Model file for the job. Use its own axes, mm. A direction names the side the tool comes from. Give positions to 0.01 mm unless a question says otherwise; leave off trailing zeros. Loops run counter-clockwise (first coordinate to the right, second up) from the corner with the lowest first, then second, coordinate; pieces in that order, holes last. Notation, with made-up numbers: (-31.75, 42.25) - (-13.75, 42.25) arc R32 ccw to (-13.75, 79.25) - close; hole circle Ø10 at (75.5, 13). An arc over 180 degrees is marked (long way). Use a Markdown table: item, result.
from build123d import *

# Parameters (mm, degrees)
SKETCH1_W           = 57.15
SKETCH1_H           = 57.15
SKETCH1_W_2         = 44.45
SKETCH1_H_2         = 44.45
BOSS_EXTRUDE1_DEPTH = 457.2
SKETCH2_W           = 44.45
SKETCH2_H           = 6.35
BOSS_EXTRUDE2_DEPTH = 44.45
SKETCH3_R           = 12.7
CUT_EXTRUDE1_DEPTH  = 6.35


with BuildPart() as part:
    # Sketch1 → Boss-Extrude1 (new body)
    with BuildSketch(Plane.XY):
        Rectangle(SKETCH1_W, SKETCH1_H)
        Rectangle(SKETCH1_W_2, SKETCH1_H_2, mode=Mode.SUBTRACT)
    extrude(amount=BOSS_EXTRUDE1_DEPTH)

    # Sketch2 → Boss-Extrude2 (add)
    with BuildSketch(Plane(origin=(0, -22.225, 0), x_dir=(1, 0, 0), z_dir=(0, 1, 0))):
        with Locations((0, -3.175)):
            Rectangle(SKETCH2_W, SKETCH2_H)
    extrude(amount=BOSS_EXTRUDE2_DEPTH)

    # Sketch3 → Cut-Extrude1 (cut)
    with BuildSketch(Plane(origin=(0, 28.575, 0), x_dir=(0, 0, -1), z_dir=(0, 1, 0))):
        with Locations(Location((-25.4, 0, 0), (0, 0, 180))):
            Circle(SKETCH3_R)
    extrude(amount=-CUT_EXTRUDE1_DEPTH, mode=Mode.SUBTRACT)


solid = part.part
(1) Pin check, flat tip, straight feed: P1, Ø3, axis at x = -9, y = -3.5, coming from the +Z side. Stop position of the tip, or through.
Computed:
| item | result |
|---|---|
| P1 | z = 6.35 |
(2) Slice it at B-B, the plane x = 0. Write the cut outline in (y, z) (3 decimals).
Computed:
| item | result |
|---|---|
| outline | (-28.575, 0) - (28.575, 0) - (28.575, 12.7) - (22.225, 12.7) - (22.225, 6.35) - (-22.225, 6.35) - (-22.225, 457.2) - (-28.575, 457.2) - close; (22.225, 38.1) - (28.575, 38.1) - (28.575, 457.2) - (22.225, 457.2) - close |
(3) Drill centre lines: probe 1 along Y at (x, z) = (20.5, 105.5) (3 decimals); probe 2 along X at (y, z) = (26.75, 25.4) (3 decimals). Where is each one in solid material? Low to high. Write a range as [from, to].
Computed:
| item | result |
|---|---|
| probe 1 | [-28.575, -22.225], [22.225, 28.575] |
| probe 2 | [-28.575, -12.7], [12.7, 28.575] |
(4) Slice it at C-C, the plane x = -17.5. Write the cut outline in (y, z) (3 decimals), plus the area to 3 significant figures.
Computed:
| item | result |
|---|---|
| outline | (-28.575, 0) - (28.575, 0) - (28.575, 457.2) - (22.225, 457.2) - (22.225, 6.35) - (-22.225, 6.35) - (-22.225, 457.2) - (-28.575, 457.2) - close |
| area | 6,090 mm² |
(5) Mould opens along X. For faces 4 (the flat face through (22.225, 0, 229)), 5 (the flat face through (28.575, 0, 225)), 6 (the flat face through (-26, 0, 457.2)) say: pulls with the +X half, pulls with the -X half, needs draft (parallel to the pull), parting line crosses it, or undercut.
Computed:
| item | result |
|---|---|
| face 4 | undercut |
| face 5 | pulls with the +X half |
| face 6 | needs draft |
(6) 3-axis set-ups, long thin cutter, end or side, ignore diameter. For faces 1 (the flat face through (0, 22.225, 229)), 2 (the flat face through (0, 0, 0)), 3 (the cylindrical face through (0.558, 25.444, 12.712)): which of +Z, -Z, +X, -X, +Y, -Y reach the whole face in a straight line?
Computed:
| item | result |
|---|---|
| face 1 | +Z |
| face 2 | -Z, +X, -X, +Y, -Y |
| face 3 | +Y |
(7) Slice it at A-A, the plane z = 114.5. Write the cut outline in (x, y) (3 decimals), plus the area to 3 significant figures.
Computed:
| item | result |
|---|---|
| outline | (-28.575, -28.575) - (28.575, -28.575) - (28.575, 28.575) - (-28.575, 28.575) - close; hole (-22.225, -22.225) - (22.225, -22.225) - (22.225, 22.225) - (-22.225, 22.225) - close |
| area | 1,290 mm² |
